Part model, mm, in its own coordinate system. A direction names the side the tool comes from. Give positions to 0.01 mm unless a question says otherwise; leave off trailing zeros. Order: outer loops, then holes, each group sorted by start corner. A loop starts at its lowest first (then second) coordinate and runs counter-clockwise, first axis right, second up. Notation, with made-up numbers: (-26, -24) - (-16, -24) arc R20 ccw to (-16, 11) - close; hole circle Ø8 at (-6, -36). An arc over 180 degrees is marked (long way). One line per item, written item: value.
```python
from build123d import *

# Parameters (mm, degrees)
SKETCH1_R           = 12.25
BOSS_EXTRUDE1_DEPTH = 1.5
SKETCH4_W           = 37
SKETCH4_H           = 1.5
BOSS_EXTRUDE2_DEPTH = 21.5
SKETCH6_R           = 1.5
CUT_EXTRUDE2_DEPTH  = 10
SKETCH3_R           = 1.6
CUT_EXTRUDE3_DEPTH  = 10
CIRPATTERN1_COUNT   = 6


with BuildPart() as part:
    # Sketch1 → Boss-Extrude1 (new body)
    with BuildSketch(Plane(origin=(0, 0, 0), x_dir=(1, 0, 0), z_dir=(0, 1, 0))):
        with BuildLine():
            Line((-23.391313752, 9.062201448), (-23.391313752, -11.937798552))
            Line((-23.391313752, -11.937798552), (13.608686248, -11.937798552))
            Line((13.608686248, -11.937798552), (13.608686248, 9.062201448))
            ThreePointArc((13.608686248, 9.062201448), (-4.891313752, 27.562201448), (-23.391313752, 9.062201448))
        make_face()
        with Locations(Location((-4.891313752, 9.062201448, 0), (0, 0, 270))):
            Circle(SKETCH1_R, mode=Mode.SUBTRACT)
    extrude(amount=BOSS_EXTRUDE1_DEPTH)

    # Sketch4 → Boss-Extrude2 (add)
    with BuildSketch(Plane(origin=(0, 1.5, 0), x_dir=(1, 0, 0), z_dir=(0, 1, 0))):
        with Locations((-4.891313752, -11.187798552)):
            Rectangle(SKETCH4_W, SKETCH4_H)
    extrude(amount=BOSS_EXTRUDE2_DEPTH)

    # Sketch6 → Cut-Extrude2 (cut)
    with BuildSketch(Plane(origin=(0, 0, 10.437798552), x_dir=(-1, 0, 0), z_dir=(0, 0, -1))):
        with Locations((-10.573464155, 6.27963227)):
            Circle(SKETCH6_R)
        with Locations((20.356091659, 6.27963227)):
            Circle(SKETCH6_R)
        with Locations((20.356091659, 18.22036773)):
            Circle(SKETCH6_R)
        with Locations((-10.573464155, 18.22036773)):
            Circle(SKETCH6_R)
    extrude(amount=-CUT_EXTRUDE2_DEPTH, mode=Mode.SUBTRACT)

    # Sketch3 → Cut-Extrude3 (cut)
    with BuildSketch(Plane(origin=(0, 1.5, 0), x_dir=(1, 0, 0), z_dir=(0, 1, 0))):
        with Locations(Location((-4.891313752, 23.562201448, 0), (0, 0, 270))):
            Circle(SKETCH3_R)
    cut_extrude3 = extrude(amount=-CUT_EXTRUDE3_DEPTH, mode=Mode.SUBTRACT)

    # CirPattern1: Cut-Extrude3 ×6 about axis
    cirpattern1_axis = Axis((-4.891313752, 0, -9.062201448), (0, 1, 0))
    for i in range(1, CIRPATTERN1_COUNT):
        add(cut_extrude3.rotate(cirpattern1_axis, i * 360 / CIRPATTERN1_COUNT), mode=Mode.SUBTRACT)


solid = part.part
```
1) Slice it at D-D on x = -20. Write the cut outline in (y, z).
Answer:
outline: (0, -19.74) - (1.5, -19.74) - (1.5, 10.44) - (4.82, 10.44) - (4.82, 11.94) - (0, 11.94) - close; (7.74, 10.44) - (16.76, 10.44) - (16.76, 11.94) - (7.74, 11.94) - close; (19.68, 10.44) - (23, 10.44) - (23, 11.94) - (19.68, 11.94) - close
2) Two-plate mould, pull along Y, no slides. Class faces 3 (the face through (-5, 12, 10.438)), 4 (the face through (11.679, 19.234, 11.177)), 5 (the face through (-5, 23, 11)), 6 (the face through (-13, 0, 1)): pulls with the +Y half, pulls with the -Y half, needs draft (parallel to the pull), parting line crosses it, or undercut.
Answer:
face 3: needs draft
face 4: undercut
face 5: pulls with the +Y half
face 6: pulls with the -Y half
3) Slice it at B-B on y = 19. Write the cut outline in (x, z).
Answer:
outline: (-23.39, 10.44) - (-21.64, 10.44) - (-21.64, 11.94) - (-23.39, 11.94) - close; (-19.07, 10.44) - (9.29, 10.44) - (9.29, 11.94) - (-19.07, 11.94) - close; (11.85, 10.44) - (13.61, 10.44) - (13.61, 11.94) - (11.85, 11.94) - close
4) Drop flat-ended pins along their axis: P1, Ø10, axis at x = -15.5, z = -12.5, coming from the +Y side; P2, Ø5, axis at x = 10.57, y = 18.22, coming from the -Z side. Give the stop position or say it passes through.
Answer:
P1: stops at y = 1.5
P2: stops at z = 10.44
5) Slice it at A-A on x = -15. Write the cut outline in (y, z).
Answer:
outline: (0, -24.56) - (1.5, -24.56) - (1.5, -15.98) - (0, -15.98) - close; (0, -2.14) - (1.5, -2.14) - (1.5, 10.44) - (23, 10.44) - (23, 11.94) - (0, 11.94) - close
6) Slice it at C-C on z = -8.5. Write the cut outline in (x, y).
Answer:
outline: (-23.39, 0) - (-17.13, 0) - (-17.13, 1.5) - (-23.39, 1.5) - close; (7.35, 0) - (13.61, 0) - (13.61, 1.5) - (7.35, 1.5) - close
7) Which spindle directions (+Z, -Z, +X, -X, +Y, -Y) get a long thin tool onto all of the face, cutting with end or side? Do faces 1 (the face through (-1.21, 0.74, 2.62)), 2 (the face through (-1, 1.5, 4)). Say none if no direction does.
Answer:
face 1: +Y, -Y
face 2: -Z, +X, -X, +Y
8) Wall check: line 1 along Z through (x, y) = (8, 16); line 2 along Y through (x, z) = (8.5, 7.5). Give the ranges that are in metal, low to high. Write a range as [from, to].
Answer:
line 1: z = [10.44, 11.94]
line 2: y = [0, 1.5]
